For this review, use the dimensioned drawing (mm, ordinates from the lowest corner) and the shaded views. Give positions to 0.01 mm unless a question says otherwise; leave off trailing zeros. Order: outer loops, then holes, each group sorted by start corner. A loop starts at its lowest first (then second) coordinate and runs counter-clockwise, first axis right, second up. Notation, with made-up numbers: M 29,-7 L 73,-7 A24 cw 73,17 Z; hole C 21,-33 d4. An arc over 180 degrees is marked long. Answer as CSV lines item,"result". Start each with the question number.
1. For line 1 along Z through (x, y) = (75.5, 5.5) (1 decimal); line 2 along Z through (x, y) = (84, 16.5) (1 decimal); line 3 along Z through (x, y) = (99, 14), list the stretches that pass through material, from the lowest coordinate up.
2. We need section A-A, the plane z = 61.5. State how many separate pieces and enclosed holes the cut face has, and give its area (3 significant figures).
3. Clearance check with flat-ended pins moving along their axes: P1, Ø1.5, axis at y = 6, z = 170, coming from the -X side; P2, Ø1.5, axis at x = 156.5, y = 11, coming from the +Z side; P3, Ø4, axis at x = 86.36, z = 152.39, coming from the +Y side; P4, Ø4, axis at y = 9, z = 150, coming from the -X side. State where each tip first meets the part, or that it passes through.
4. Mouldability with a two-part tool opening along Z and no side actions: class the marked faces 1, 2 and 3 as pulls with the +Z half, pulls with the -Z half, needs draft (parallel to the pull), parting line crosses it, or undercut.
5. We need section B-B, the plane z = 161. Give the boundary of the cut face in (x, y).
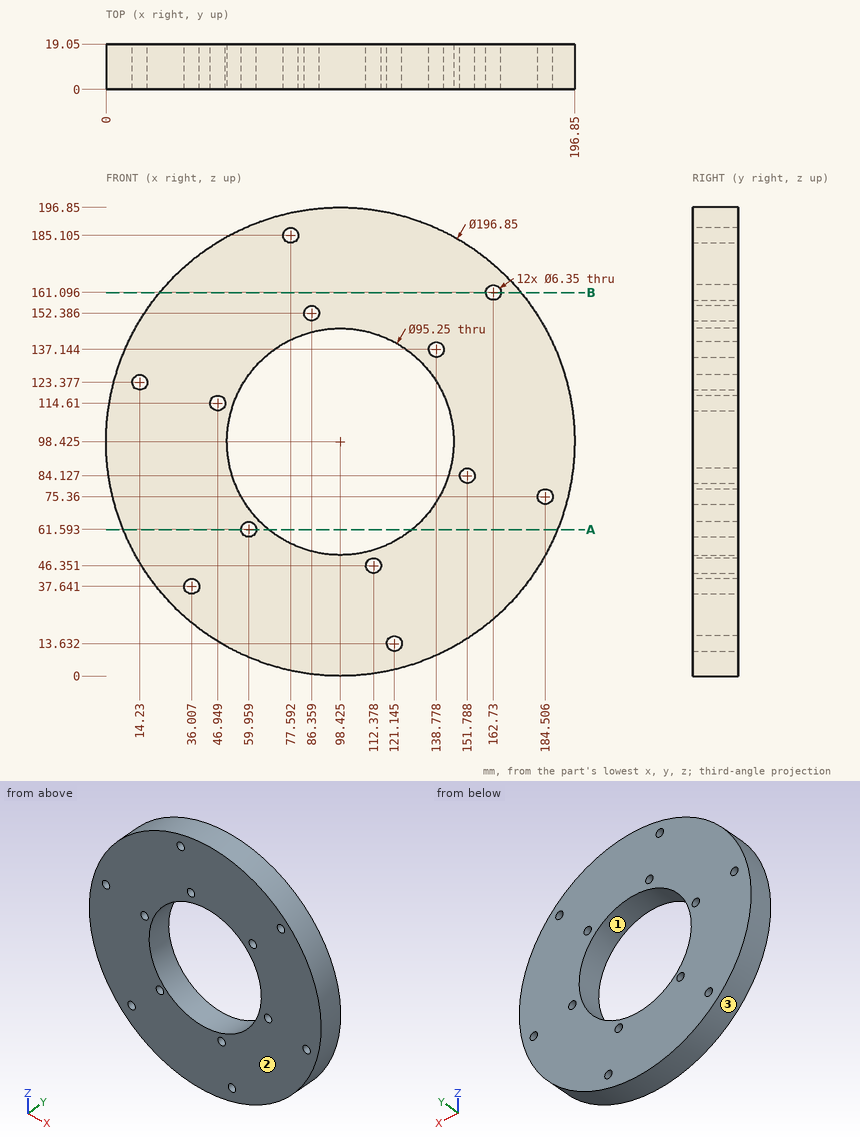
Result set:
1,line 1,"2.7 to 56.7, 140.2 to 182.7, 187.5 to 194.1"
1,line 2,"1.1 to 53, 143.8 to 150.3, 154.5 to 195.8"
1,line 3,"0 to 50.8, 146.05 to 196.85"
2,separate pieces,"3"
2,enclosed holes,"0"
2,area,"2,210 mm2"
3,P1,"x = 30.08"
3,P2,"z = 178.43"
3,P3,"through"
3,P4,"x = 13.4"
4,face 1,"undercut"
4,face 2,"needs draft"
4,face 3,"parting line crosses it"
5,outline,"M 22.45,0 L 159.56,0 L 159.56,19.05 L 22.45,19.05 Z; M 165.9,0 L 174.4,0 L 174.4,19.05 L 165.9,19.05 Z"
